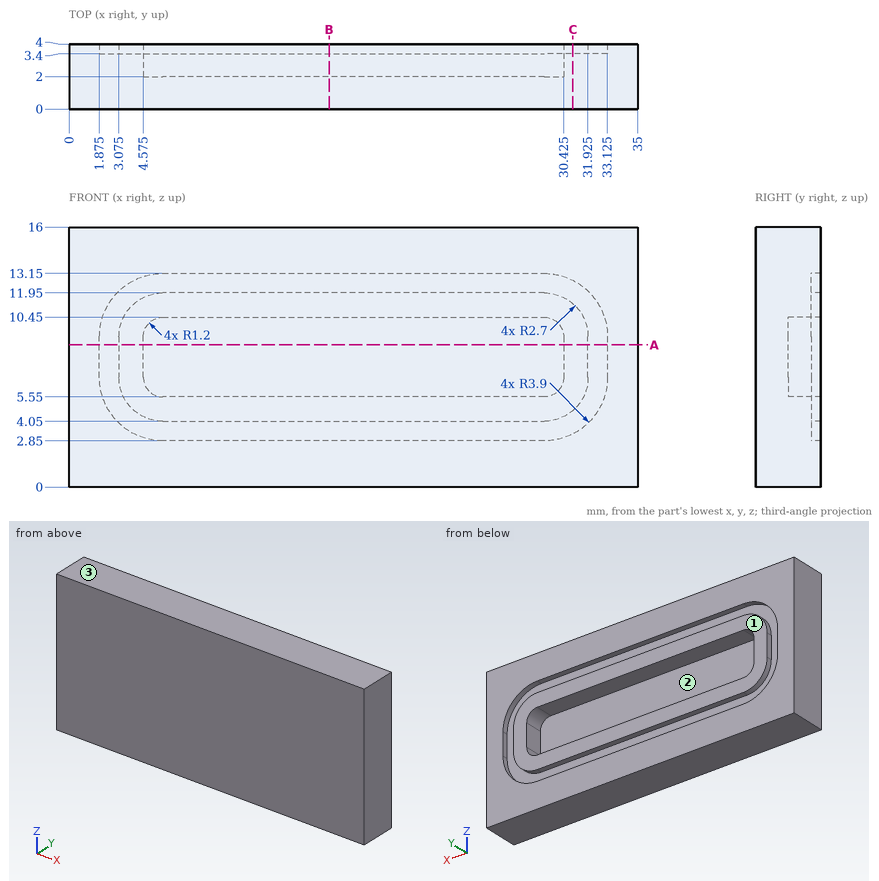
Print and shaded views of the part. All mm, measured from the part's lowest x, y and z. Coordinates: 2 decimals unless noted, no trailing zeros. Write each loop counter-clockwise with the first axis right and the second up, starting at its lowest first coordinate (ties: lowest second). Pieces come first, ordered by that corner, then holes.
(1) Flat gauge pin, fed straight in: pin 1 (5 mm diameter, centred on x = 4.5, z = 9, fed in from -Y). Where does the tip first touch, or does it go through?
(2) Two-plate mould, pull along Z, no slides. Class the marked faces 1, 2 and 3: +Z half, -Z half, draft (parallel to the pull), parting line (faces both ways), or undercut.
(3) Cut at A-A, the plane z = 8.75. List the corners of the cut face in (x, y) (3 decimals).
(4) Drill centre lines: probe 1 along Z at (x, y) = (18.5, 3.6); probe 2 along Z at (x, y) = (14, 3); probe 3 along Y at (x, z) = (24, 9.25). Where is each one in solid material? Low to high.
(5) Cut at B-B, the plane x = 16. List the corners of the cut face in (y, z).
(6) Cut at C-C, the plane x = 31. List the corners of the cut face in (y, z).
Geometry says:
1. pin 1: stops at y = 0
2. face 1: draft
2. face 2: undercut
2. face 3: +Z half
3. outline: (0, 0) - (35, 0) - (35, 4) - (33.125, 4) - (33.125, 3.4) - (31.925, 3.4) - (31.925, 4) - (30.425, 4) - (30.425, 2) - (4.575, 2) - (4.575, 4) - (3.075, 4) - (3.075, 3.4) - (1.875, 3.4) - (1.875, 4) - (0, 4) - close
4. probe 1: z = 0 to 2.85, 4.05 to 5.55, 10.45 to 11.95, 13.15 to 16
4. probe 2: z = 0 to 5.55, 10.45 to 16
4. probe 3: y = 0 to 2
5. outline: (0, 0) - (4, 0) - (4, 2.85) - (3.4, 2.85) - (3.4, 4.05) - (4, 4.05) - (4, 5.55) - (2, 5.55) - (2, 10.45) - (4, 10.45) - (4, 11.95) - (3.4, 11.95) - (3.4, 13.15) - (4, 13.15) - (4, 16) - (0, 16) - close
6. outline: (0, 0) - (4, 0) - (4, 3.28) - (3.4, 3.28) - (3.4, 4.72) - (4, 4.72) - (4, 11.28) - (3.4, 11.28) - (3.4, 12.72) - (4, 12.72) - (4, 16) - (0, 16) - close
